```python
from build123d import *

# Parameters (mm, degrees)
F1_DEPTH = 50
F2_R     = 60
F3_DEPTH = 12


with BuildPart() as f1:
    # F0 (on Front) → F1 (new body, symmetric)
    with BuildSketch(Plane.XZ):
        Polygon((-12, 65), (0, 65), (12, 65), (12, -6), (15, -6), (15, 68), (0, 68), (-15, 68), (-15, -6), (-12, -6), align=None)
    extrude(amount=F1_DEPTH, both=True)

    # F2 (on Right) → F3 (join, symmetric)
    with BuildSketch(Plane.YZ):
        Circle(F2_R)
    extrude(amount=F3_DEPTH, both=True)


solid = f1.part
```
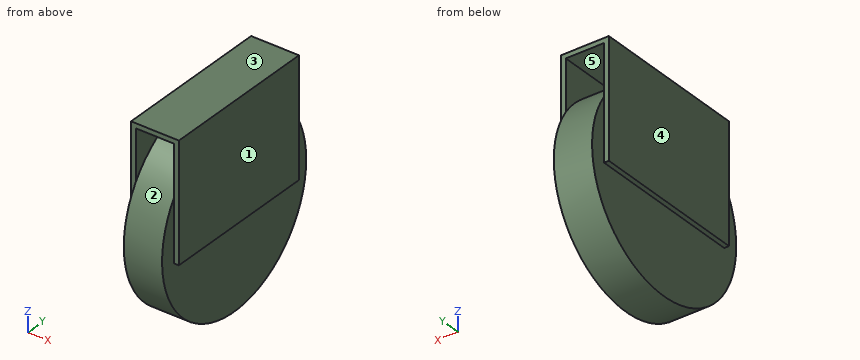
Build history of the part. All positions in model axes, mm. Face numbers are marked on the shaded views. A direction names the side the tool comes from. Give positions to 0.01 mm unless a question says otherwise; leave off trailing zeros. Loops run counter-clockwise (first coordinate to the right, second up) from the corner with the lowest first, then second, coordinate; pieces in that order, holes last.
1) Band-saw the part on D-D on y = -23.5. List the corners of the cut face in (x, z), then the cut area to 3 significant figures.
Values follow:
outline: (-15, -6) - (-12, -6) - (-12, -55.21) - (12, -55.21) - (12, -6) - (15, -6) - (15, 68) - (-15, 68) - close; hole (-12, 55.21) - (12, 55.21) - (12, 65) - (-12, 65) - close
area: 3,170 mm2
2) Band-saw the part on C-C on z = 28. List the corners of the cut face in (x, y), then the cut area to 3 significant figures.
Values follow:
outline: (-15, -50) - (-12, -50) - (-12, -53.07) - (12, -53.07) - (12, -50) - (15, -50) - (15, 50) - (12, 50) - (12, 53.07) - (-12, 53.07) - (-12, 50) - (-15, 50) - close
area: 3,150 mm2
3) Band-saw the part on A-A on x = -2.75. List the corners of the cut face in (y, z), then the cut area to 3 significant figures.
Values follow:
outline: circle Ø120 at (0, 0); (-50, 65) - (50, 65) - (50, 68) - (-50, 68) - close
area: 11,600 mm2
4) 3-axis set-ups, long thin cutter, end or side, ignore diameter. For the marked faces 1 and 2: which of +Z, -Z, +X, -X, +Y, -Y reach the whole face in a straight line?
Values follow:
face 1: +Z, -Z, +X, +Y, -Y
face 2: none
5) Probe line 1 along X through (y, z) = (45, 61); line 2 along Z through (x, y) = (1.25, 47.5); line 3 along X through (y, z) = (-3.5, -43). List the from-to ranges inside material, lowest first.
Values follow:
line 1: x = -15 to -12, 12 to 15
line 2: z = -36.66 to 36.66, 65 to 68
line 3: x = -12 to 12
6) Two-plate mould, pull along Z, no slides. Class the marked faces 3, 4 and 5: released by +Z, released by -Z, zero draft, split by the parting line, or undercut.
Values follow:
face 3: released by +Z
face 4: zero draft
face 5: undercut
7) Drop flat-ended pins along their axis: P1, Ø9, axis at x = -3, z = 43, coming from the +Y side; P2, Ø8, axis at x = 7, z = -23.5, coming from the +Y side; P3, Ø10, axis at y = 34, z = -20, coming from the -X side. Give the stop position or say it passes through.
Values follow:
P1: stops at y = 46.02
P2: stops at y = 56.74
P3: stops at x = -12
8) Band-saw the part on B-B on y = 0. List the corners of the cut face in (x, z), then the cut area to 3 significant figures.
Values follow:
outline: (-15, -6) - (-12, -6) - (-12, -60) - (12, -60) - (12, -6) - (15, -6) - (15, 68) - (-15, 68) - close; hole (-12, 60) - (12, 60) - (12, 65) - (-12, 65) - close
area: 3,400 mm2
